Geometry check sheet. Reference: the model listing, model coordinates, mm. Face numbers are marked on the shaded views. A direction names the side the tool comes from. Coordinates: 2 decimals unless noted, no trailing zeros. Loops run counter-clockwise (first coordinate to the right, second up) from the corner with the lowest first, then second, coordinate; pieces in that order, holes last. Notation, with made-up numbers: (6, 39.25) - (55, 39.25) arc R34 cw to (55, 78.25) - close; hole circle Ø2 at (69, -35.5). An arc over 180 degrees is marked (long way). Write item = value, one per line. Start each with the question number.
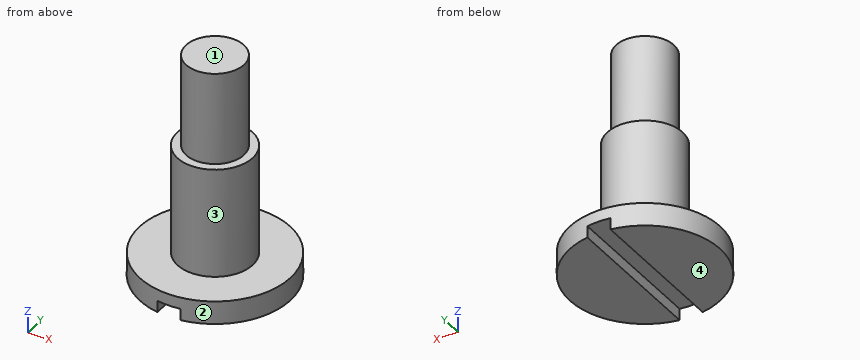
Autodesk Inventor part; units mm, degrees
ref_plane "Work Plane1" through (0, 6.5, 0) normal (0, 1, 0) x (-1, 0, 0)
ref_plane "YZ Plane" through (0, 0, 0) normal (1, 0, 0) x (0, 1, 0)
ref_plane "XY Plane" through (0, 0, 0) normal (0, 0, 1) x (1, 0, 0)
sketch "Sketch1" plane through (0, 0, 0) normal (0, 0, 1) x (1, 0, 0)
  circle A0 centre (0, 0) radius 6.5
  dimension "d0" = 13
extrude "Extrusion1" add sketch "Sketch1" along normal blind 2
sketch "Sketch2" plane through (0, 0, 2) normal (0, 0, 1) x (1, 0, 0)
  circle A0 centre (0, 0) radius 6.5
  circle A1 centre (0, 0) radius 3.25
  dimension "d3" = 6.5
extrude "Extrusion2" add sketch "Sketch2" along normal blind 9.5 contours A1
ref_plane "Work Plane1" through (0, 6.5, 0) normal (0, 1, 0) x (-1, 0, 0)
sketch "Sketch3" plane through (0, 6.5, 0) normal (0, 1, 0) x (-1, 0, 0)
  line L0 (6.5, 0) -> (-6.5, 0)
  line L1 (-1, 0) -> (1, 0)
  line L2 (1, 0) -> (1, 1)
  line L3 (1, 1) -> (-1, 1)
  line L4 (-1, 1) -> (-1, 0)
  point P0 (0, 0)
  point P1 (1, 0.5)
  point P2 (0, 0)
  dimension "d7" = 2
  dimension "d8" = 1
  dimension "d9" = 1
extrude "Extrusion3" cut sketch "Sketch3" against normal through all
sketch "Sketch4" plane through (0, 0, 11.5) normal (0, 0, 1) x (1, 0, 0)
  circle A0 centre (0, 0) radius 3.25
  circle A1 centre (0, 0) radius 2.5
  dimension "d12" = 5
extrude "Extrusion4" add sketch "Sketch4" along normal blind 8 contours A1
thread "Thread1"
properties part number "Crankpin" material "Steel AISI 1020 107 HR"
(1) Tool access check on the marked faces 3 and 4. Record the directions out of +Z, -Z, +X, -X, +Y, -Y that give a thin tool (end or side, any length) a straight path to the whole face; none if there is none.
(2) Scan lines: line 1 (Z direction, x = 0.75, y = 2); line 2 (Z direction, x = -0.25, y = 3.75); line 3 (X direction, y = 2, z = 12.75). Record each from-to range of solid material in increasing order.
(3) Depth check by flat-ended pin: pin 1 (0.5 mm diameter, centred on y = -2.5, z = 0.5, fed in from -X); pin 2 (6 mm diameter, centred on y = -0.5, z = 10.5, fed in from +X); pin 3 (1.5 mm diameter, centred on x = -1, z = 7, fed in from -Y). Enter the tip coordinate at first touch or a pass-through.
(4) Sectioned sample at C-C on z = 12. Enter the section's corners in (x, y), plus the area to 3 significant figures.
(5) Sectioned sample at B-B on x = 0. Enter the section's corners in (y, z), plus the area to 3 significant figures.
(6) Draft check along X on the marked faces 1 and 2. Enter one of: pulls with the +X half, pulls with the -X half, needs draft (parallel to the pull), parting line crosses it, or undercut.
(7) Sectioned sample at D-D on y = 3. Enter the section's corners in (x, z).
(8) Sectioned sample at A-A on y = 0. Enter the section's corners in (x, z).
Working result:
q1.face_3 = +Z
q1.face_4 = -Z, +X, -X, +Y, -Y
q2.line_1 = 1 to 19.5
q2.line_2 = 1 to 2
q2.line_3 = -1.5 to 1.5
q3.pin_1 = -6.1
q3.pin_2 = 3.25
q3.pin_3 = -3.24
q4.outline = circle Ø5 at (0, 0)
q4.area = 19.6 mm2
q5.outline = (-6.5, 1) - (6.5, 1) - (6.5, 2) - (3.25, 2) - (3.25, 11.5) - (2.5, 11.5) - (2.5, 19.5) - (-2.5, 19.5) - (-2.5, 11.5) - (-3.25, 11.5) - (-3.25, 2) - (-6.5, 2) - close
q5.area = 115 mm2
q6.face_1 = needs draft
q6.face_2 = parting line crosses it
q7.outline = (-5.77, 0) - (-1, 0) - (-1, 1) - (1, 1) - (1, 0) - (5.77, 0) - (5.77, 2) - (1.25, 2) - (1.25, 11.5) - (-1.25, 11.5) - (-1.25, 2) - (-5.77, 2) - close
q8.outline = (-6.5, 0) - (-1, 0) - (-1, 1) - (1, 1) - (1, 0) - (6.5, 0) - (6.5, 2) - (3.25, 2) - (3.25, 11.5) - (2.5, 11.5) - (2.5, 19.5) - (-2.5, 19.5) - (-2.5, 11.5) - (-3.25, 11.5) - (-3.25, 2) - (-6.5, 2) - close
